Geometry check sheet. Reference: the model listing, model coordinates, mm. Round coordinates to 2 decimals unless told otherwise and drop trailing zeros. Write each loop counter-clockwise with the first axis right and the second up, starting at its lowest first coordinate (ties: lowest second). Pieces come first, ordered by that corner, then holes. Notation, with made-up numbers: M -10,19 L 9,19 A9 cw 9,26 Z; hole C 59.25,34 d11. An arc over 180 degrees is marked long. Use a Markdown table: item, result.
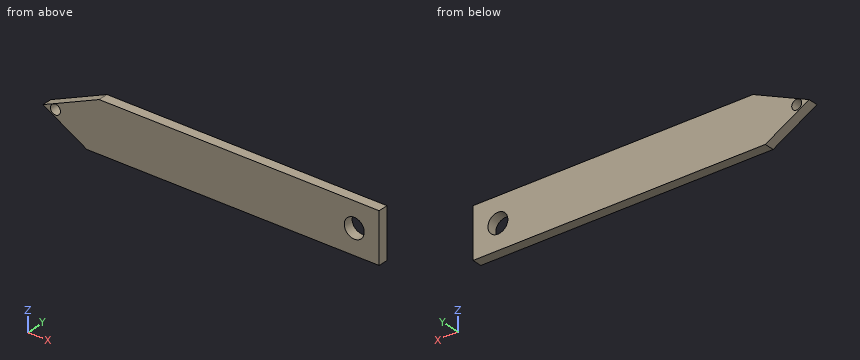
```python
from build123d import *

# Parameters (mm, degrees)
SKETCH1_W           = 67.5
SKETCH1_H           = 10
SKETCH1_R           = 1
SKETCH1_R_2         = 2
BOSS_EXTRUDE1_DEPTH = 2
FILLET2_R           = 5
FILLET3_R           = 5
CUT_EXTRUDE1_DEPTH  = 10


with BuildPart() as part:
    # Sketch1 → Boss-Extrude1 (new body)
    with BuildSketch(Plane(origin=(0, 0, 0), x_dir=(1, 0, 0), z_dir=(0, 1, 0))):
        with Locations((7.54504806, 0.629386767)):
            Rectangle(SKETCH1_W, SKETCH1_H)
        with Locations(Location((-23.70495194, 0.629386767, 0), (0, 0, 270))):
            Circle(SKETCH1_R, mode=Mode.SUBTRACT)
        with Locations(Location((36.29504806, 0.629386767, 0), (0, 0, 270))):
            Circle(SKETCH1_R_2, mode=Mode.SUBTRACT)
    extrude(amount=BOSS_EXTRUDE1_DEPTH)

    # Fillet2
    fillet2_edges = [part.edges().sort_by_distance(p)[0] for p in [
        (-26.20495194, 1, -5.629386767),
    ]]
    fillet(fillet2_edges, radius=FILLET2_R)

    # Fillet3
    fillet3_edges = [part.edges().sort_by_distance(p)[0] for p in [
        (-26.20495194, 1, 4.370613233),
    ]]
    fillet(fillet3_edges, radius=FILLET3_R - 0.0001)  # a hair under: the kernel refuses the full size

    # Sketch2 → Cut-Extrude1 (cut)
    with BuildSketch(Plane(origin=(0, 2, 0), x_dir=(1, 0, 0), z_dir=(0, 1, 0))):
        Polygon((-26.20495194, 0.629386767), (-17.3953026, 5.629386767), (-30.276307772, 5.629386767), (-27.957364893, -6.288007195), (-14.932537807, -4.370613233), align=None)
    extrude(amount=-CUT_EXTRUDE1_DEPTH, mode=Mode.SUBTRACT)


solid = part.part
```
Item 1: Material ranges on line 1 along X through (y, z) = (1.55, -1.5); line 2 along X through (y, z) = (1.8, 1); line 3 along X through (y, z) = (1.4, 0), recorded low to high. Write a range as from..to.
Outcome:
| item | result |
|---|---|
| line 1 | x = -24.67..-24.2, -23.21..34.49, 38.1..41.3 |
| line 2 | x = -22.53..35.14, 37.45..41.3 |
| line 3 | x = -24.79..-24.48, -22.93..34.4, 38.19..41.3 |
Item 2: Cross-section at B-B, the plane x = -21.5. Record the cut outline in (y, z), and give its area (3 significant figures).
Outcome:
| item | result |
|---|---|
| outline | M 0,-3.3 L 2,-3.3 L 2,1.46 L 0,1.46 Z |
| area | 9.51 mm2 |
Item 3: Cross-section at A-A, the plane y = 0.95. Record the cut outline in (x, z), and give its area (3 significant figures).
Outcome:
| item | result |
|---|---|
| outline | M -26.2,-0.63 L -17.4,-5.63 L 41.3,-5.63 L 41.3,4.37 L -14.93,4.37 Z; hole C -23.7,-0.63 d2; hole C 36.3,-0.63 d4 |
| area | 609 mm2 |
